Verification items for the finished model (mm, model axes). Face numbers are marked on the shaded views. A direction names the side the tool comes from. Round coordinates to 2 decimals unless told otherwise and drop trailing zeros. Loops run counter-clockwise (first coordinate to the right, second up) from the corner with the lowest first, then second, coordinate; pieces in that order, holes last. Notation, with made-up numbers: (80.5, 37.25) -> (120.5, 37.25) arc R12 ccw to (120.5, 55.25) -> close; hole circle Ø7 at (64, 2). An arc over 180 degrees is marked (long way). Write item = value, one per line. Start each with the question number.
```python
from build123d import *

# Parameters (mm, degrees)
F0_W     = 40
F0_H     = 22.2
F0_R     = 2.125
F0_R_2   = 7.825
F1_DEPTH = 5
F2_R     = 11.1
F2_R_2   = 7.825
F3_DEPTH = 19.5
F4_R     = 11.1
F4_R_2   = 4.75
F5_DEPTH = 5
F6_R     = 11.09999
F7_R     = 2.5
F8_R     = 5
F9_DEPTH = 4


# Not quite as in the source:
# - a fillet or chamfer is up to 0.001 mm smaller than in the source, because OpenCascade refuses the exact size


with BuildPart() as f1:
    # F0 (on Top) → F1 (new body)
    with BuildSketch(Plane.XY):
        Rectangle(F0_W, F0_H)
        with Locations((-15, 0)):
            Circle(F0_R, mode=Mode.SUBTRACT)
        Circle(F0_R_2, mode=Mode.SUBTRACT)
        with Locations((15, 0)):
            Circle(F0_R, mode=Mode.SUBTRACT)
    extrude(amount=F1_DEPTH)

    # F2 (on face) → F3 (join)
    with BuildSketch(Plane.XY.offset(5)):
        Circle(F2_R)
        Circle(F2_R_2, mode=Mode.SUBTRACT)
    extrude(amount=F3_DEPTH)

    # F4 (on face) → F5 (join)
    with BuildSketch(Plane.XY.offset(24.5)):
        Circle(F4_R)
        Circle(F4_R_2, mode=Mode.SUBTRACT)
    extrude(amount=F5_DEPTH)

    # F6 (radius 11.1 in the source; OpenCascade refuses exactly that, so slightly less here)
    f6_edges = [f1.edges().sort_by_distance(p)[0] for p in [
        (-20, 11.1, 2.5),
        (-20, -11.1, 2.5),
        (20, -11.1, 2.5),
        (20, 11.1, 2.5),
    ]]
    fillet(f6_edges, radius=F6_R)

    # F7
    f7_edges = [f1.edges().sort_by_distance(p)[0] for p in [
        (-11.1, 0, 29.5),
    ]]
    fillet(f7_edges, radius=F7_R)

    # F8 (on face) → F9 (join)
    with BuildSketch(Plane.XY.offset(5)):
        with Locations((-15, 0)):
            Circle(F8_R)
        Polygon((-15, 3.3774990748), (-12.075, 1.6887495374), (-12.075, -1.6887495374), (-15, -3.3774990748), (-17.925, -1.6887495374), (-17.925, 1.6887495374), align=None, mode=Mode.SUBTRACT)
        with Locations((15, 0)):
            Circle(F8_R)
        Polygon((12.075, -1.6887495374), (12.075, 1.6887495374), (15, 3.3774990748), (17.925, 1.6887495374), (17.925, -1.6887495374), (15, -3.3774990748), align=None, mode=Mode.SUBTRACT)
    extrude(amount=F9_DEPTH)


solid = f1.part
```
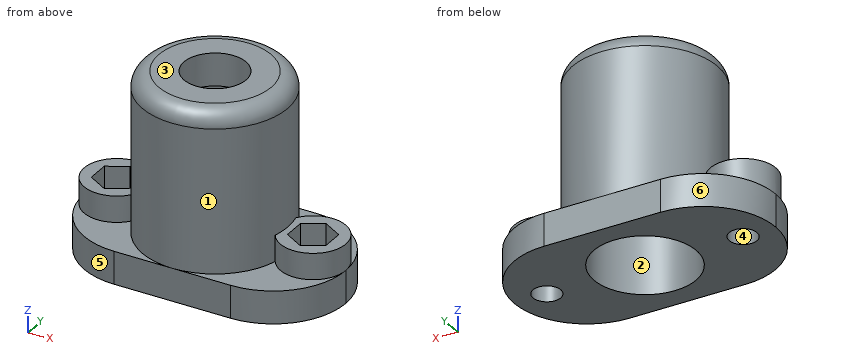
(1) Section check A-A on x = 13.5. Enter the section's corners in (y, z).
(2) Draft check along Y on the marked faces 4, 5 and 6. Enter one of: +Y half, -Y half, draft (parallel to the pull), parting line (faces both ways), or undercut.
(3) Access from +Z, -Z, +X, -X, +Y, -Y to the whole of each face (thin tool, end or side, straight path). Record for the marked faces 1, 2 and 3.
(4) Depth check by flat-ended pin: pin 1 Ø1 at (y, z) = (-0.5, 7.5) entering from -X; pin 2 Ø10 at (y, z) = (5, 17.5) entering from +X; pin 3 Ø3 at (x, y) = (-15, 2.5) entering from +Z; pin 4 Ø1.8 at (x, y) = (-15, 1.5) entering from +Z. Enter the tip coordinate at first touch or a pass-through.
(5) Section check B-B on z = 8. Give the number of separate pieces and of enclosed holes in the cut face, then the cut area to 3 significant figures.
(6) Scan lines: line 1 (Y direction, x = 0, z = 19.5) (3 decimals); line 2 (X direction, y = -3.25, z = 5.5); line 3 (Z direction, x = -14, y = -8.75). Record each from-to range of solid material in increasing order. Write a range as [from, to].
Computed values:
q1.outline = (-10.1, 0) -> (-1.51, 0) -> (-1.51, 5) -> (-2.51, 5) -> (-2.51, 9) -> (-4.77, 9) -> (-4.77, 5) -> (-10.1, 5) -> close; (1.51, 0) -> (10.1, 0) -> (10.1, 5) -> (4.77, 5) -> (4.77, 9) -> (2.51, 9) -> (2.51, 5) -> (1.51, 5) -> close
q2.face_4 = undercut
q2.face_5 = -Y half
q2.face_6 = +Y half
q3.face_1 = +Z
q3.face_2 = -Z
q3.face_3 = +Z, +X, -X, +Y, -Y
q4.pin_1 = -20
q4.pin_2 = 11.1
q4.pin_3 = 9
q4.pin_4 = 5
q5.separate_pieces = 1
q5.enclosed_holes = 3
q5.area = 285 mm²
q6.line_1 = [-11.1, -7.825], [7.825, 11.1]
q6.line_2 = [-18.8, -15.22], [-14.78, -11.2], [-10.61, -7.12], [7.12, 10.61], [11.2, 14.78], [15.22, 18.8]
q6.line_3 = [0, 5]
